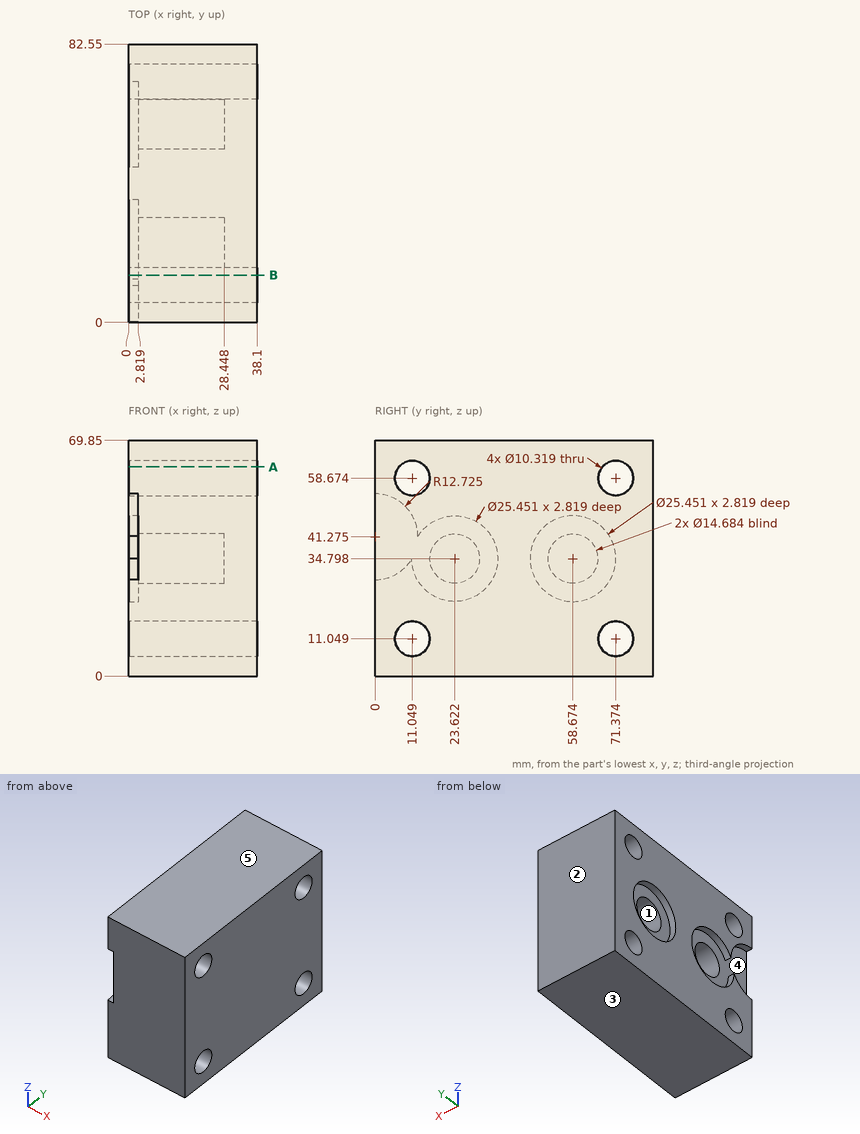
Answer from the drawing. Dimensions are ordinates in mm from the lowest x, y and z of the part. A direction names the side the tool comes from. Give positions to 0.01 mm unless a question says otherwise; leave off trailing zeros. Write each loop counter-clockwise with the first axis right and the second up, starting at its lowest first coordinate (ties: lowest second). Pieces come first, ordered by that corner, then holes. Notation, with made-up numbers: (74.25, 39) -> (121.25, 39) arc R32 ccw to (121.25, 75) -> close; hole circle Ø6 at (-39, 64.5). An arc over 180 degrees is marked (long way). Use a Markdown table: item, result.
(1) Section B-B, the plane y = 14 is taken. Determine the outline of the cut face in (x, z), then the cut area to 3 significant figures.
Return value:
| item | result |
|---|---|
| outline | (0, 0) -> (38.1, 0) -> (38.1, 6.82) -> (0, 6.82) -> close; (0, 15.28) -> (38.1, 15.28) -> (38.1, 54.44) -> (0, 54.44) -> (0, 43.13) -> (2.82, 43.13) -> (2.82, 26.47) -> (0, 26.47) -> close; (0, 62.91) -> (38.1, 62.91) -> (38.1, 69.85) -> (0, 69.85) -> close |
| area | 1,970 mm2 |
(2) For the marked faces 1 and 2, determine the directions among +Z, -Z, +X, -X, +Y, -Y from which every point of the face is accessible in a straight line to the end or side of a thin tool.
Return value:
| item | result |
|---|---|
| face 1 | -X |
| face 2 | +Z, -Z, +X, -X, +Y |
(3) Section A-A, the plane z = 62 is taken. Give the number of separate pieces and of enclosed holes in the cut face, then the cut area to 3 significant figures.
Return value:
| item | result |
|---|---|
| separate pieces | 3 |
| enclosed holes | 0 |
| area | 2,540 mm2 |
(4) Determine the mould class of the marked faces 3, 4 and 5 for opening direction Z: released by +Z, released by -Z, zero draft, split by the parting line, or undercut.
Return value:
| item | result |
|---|---|
| face 3 | released by -Z |
| face 4 | undercut |
| face 5 | released by +Z |
(5) A flat-ended cylindrical pin translates along its axis: P1, Ø8, axis at y = 62.5, z = 33.5, coming from the -X side. Find the tip coordinate at first contact, or state that the pin passes through.
Return value:
| item | result |
|---|---|
| P1 | x = 2.82 |
(6) Find the intervals of material crossed by probe 1 along Z at (x, y) = (27, 58.5); probe 2 along X at (y, z) = (66.5, 32.5), in increasing order. Write a range as from..to.
Return value:
| item | result |
|---|---|
| probe 1 | 0..27.46, 42.14..69.85 |
| probe 2 | 2.82..38.1 |
